```python
from build123d import *

# Parameters (mm, degrees)
SKETCH2_R           = 1.937236025
SKETCH2_R_2         = 1.25
BOSS_EXTRUDE2_DEPTH = 15


with BuildPart() as part:
    # Sketch2 → Boss-Extrude2 (new body)
    with BuildSketch(Plane(origin=(0, 0, 0), x_dir=(1, 0, 0), z_dir=(0, 1, 0))):
        with BuildLine():
            Line((0, 0), (20, 0))
            Line((20, 0), (20, 9))
            Line((20, 9), (0, 9))
            ThreePointArc((0, 9), (-4.5, 4.5), (0, 0))
        make_face()
        with Locations(Location((0, 4.5, 0), (0, 0, 270))):
            Circle(SKETCH2_R, mode=Mode.SUBTRACT)
        with Locations(Location((7.5, 4.5, 0), (0, 0, 270))):
            Circle(SKETCH2_R_2, mode=Mode.SUBTRACT)
        with Locations(Location((15, 4.5, 0), (0, 0, 270))):
            Circle(SKETCH2_R_2, mode=Mode.SUBTRACT)
    extrude(amount=BOSS_EXTRUDE2_DEPTH)


solid = part.part
```
Geometry: final body of the model. Coordinates: model frame, mm. Coordinates: 2 decimals unless noted, no trailing zeros. Order: outer loops, then holes, each group sorted by start corner. A loop starts at its lowest first (then second) coordinate and runs counter-clockwise, first axis right, second up. Notation, with made-up numbers: (83, -27.75) -> (115, -27.75) arc R12 ccw to (115, -23.75) -> close; hole circle Ø3 at (30, -33). An arc over 180 degrees is marked (long way). Answer in a Markdown table with one row per item.
Item 1: Section B-B on y = 11.5. Output: boundary loops of the cut face in (x, z), plus the area to 3 significant figures.
Return value:
| item | result |
|---|---|
| outline | (0, -9) -> (20, -9) -> (20, 0) -> (0, 0) arc R4.5 ccw to start; hole circle Ø3.87 at (0, -4.5); hole circle Ø2.5 at (7.5, -4.5); hole circle Ø2.5 at (15, -4.5) |
| area | 190 mm² |
Item 2: Section A-A on x = 14. Output: boundary loops of the cut face in (y, z), plus the area to 4 significant figures.
Return value:
| item | result |
|---|---|
| outline | (0, -9) -> (15, -9) -> (15, -5.25) -> (0, -5.25) -> close; (0, -3.75) -> (15, -3.75) -> (15, 0) -> (0, 0) -> close |
| area | 112.5 mm² |
Item 3: Section D-D on x = 7.5. Output: boundary loops of the cut face in (y, z).
Return value:
| item | result |
|---|---|
| outline | (0, -9) -> (15, -9) -> (15, -5.75) -> (0, -5.75) -> close; (0, -3.25) -> (15, -3.25) -> (15, 0) -> (0, 0) -> close |
Item 4: Ray query, L1, parallel to X at y = 5, z = -4.5; L2, parallel to X at y = 10, z = -4; L3, parallel to X at y = 12.75, z = -2.75. Return the intervals inside material, ascending.
Return value:
| item | result |
|---|---|
| L1 | x = -4.5 to -1.94, 1.94 to 6.25, 8.75 to 13.75, 16.25 to 20 |
| L2 | x = -4.47 to -1.87, 1.87 to 6.35, 8.65 to 13.85, 16.15 to 20 |
| L3 | x = -4.15 to -0.83, 0.83 to 20 |
Item 5: Draft query along X for faces 1 (the cylindrical face through (16.054, 7.395, -3.828)), 2 (the cylindrical face through (0.58, 7.4, -2.65)), 3 (the flat face through (20, 7, -4)), 4 (the flat face through (10, 7, -9)). Return one class per face: released by +X, released by -X, zero draft, split by the parting line, or undercut.
Return value:
| item | result |
|---|---|
| face 1 | undercut |
| face 2 | undercut |
| face 3 | released by +X |
| face 4 | zero draft |
Item 6: Section C-C on z = -4.5. Output: boundary loops of the cut face in (x, y).
Return value:
| item | result |
|---|---|
| outline | (-4.5, 0) -> (-1.94, 0) -> (-1.94, 15) -> (-4.5, 15) -> close; (1.94, 0) -> (6.25, 0) -> (6.25, 15) -> (1.94, 15) -> close; (8.75, 0) -> (13.75, 0) -> (13.75, 15) -> (8.75, 15) -> close; (16.25, 0) -> (20, 0) -> (20, 15) -> (16.25, 15) -> close |
